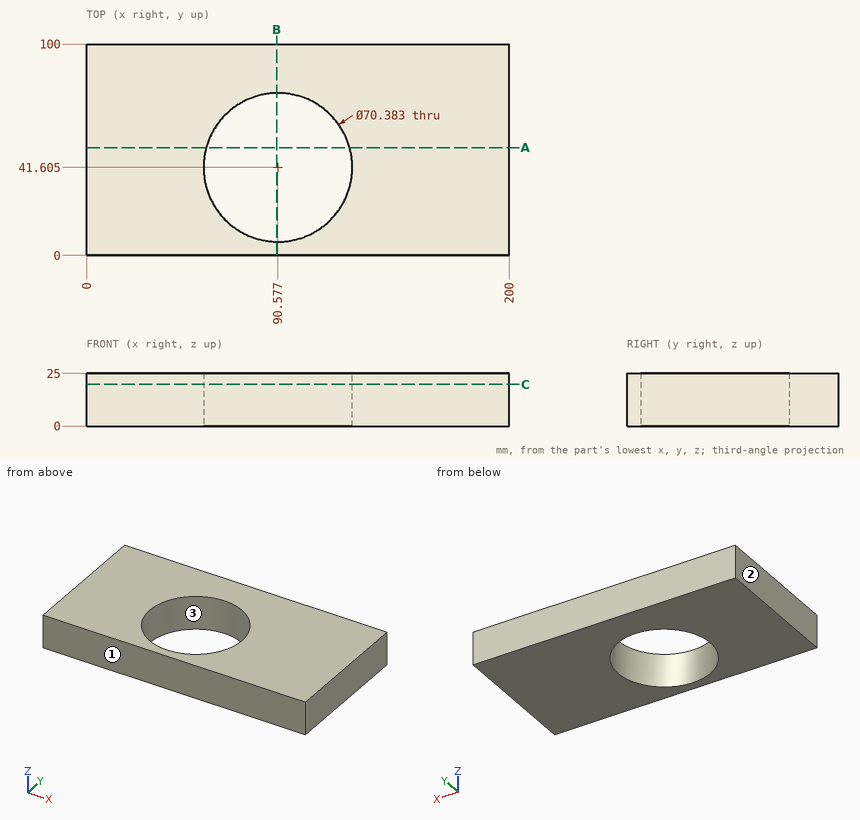
Could you check a few things on this drawing? It's one solid part, dimensions in mm from its lowest x, y, z. Give positions to 0.01 mm unless a question says otherwise; leave off trailing zeros. Order: outer loops, then holes, each group sorted by start corner. A loop starts at its lowest first (then second) coordinate and runs counter-clockwise, first axis right, second up. Notation, with made-up numbers: (34.5, -30) - (58.5, -30) arc R22 cw to (58.5, -24) - close; hole circle Ø5 at (21.5, 75.25). An arc over 180 degrees is marked (long way). One line per question, with ' | ' between items. Start each with the question number.
Item 1: I want a section at A-A on y = 51. Write out the boundary of the cut face in (x, z), then the cut area to 3 significant figures.
Item 2: I want a section at B-B on x = 90. Write out the boundary of the cut face in (y, z).
Item 3: I want a section at C-C on z = 19.75. Write out the boundary of the cut face in (x, y) (1 decimal).
Item 4: I need wall thicknesses on probe 1 along X at (y, z) = (57, 17.25); probe 2 along X at (y, z) = (16.5, 11.25) (1 decimal); probe 3 along Y at (x, z) = (118.5, 13) (1 decimal). Which ranges of each line are inside material? Lowest first, please. Write a range as [from, to].
Item 5: I'm going to push a flat-ended pin straight in: pin 1 Ø5 at (x, z) = (139.5, 5.5) entering from -Y. Where does the tip first touch, or does it pass through?
Item 6: Thinking about a two-plate mould opening in X: for the marked faces 1, 2 and 3, which applies, pulls with the +X half, pulls with the -X half, needs draft (parallel to the pull), parting line crosses it, or undercut?
Verdict:
1) outline: (0, 0) - (56.66, 0) - (56.66, 25) - (0, 25) - close; (124.49, 0) - (200, 0) - (200, 25) - (124.49, 25) - close | area: 3,300 mm^2
2) outline: (0, 0) - (6.42, 0) - (6.42, 25) - (0, 25) - close; (76.79, 0) - (100, 0) - (100, 25) - (76.79, 25) - close
3) outline: (0, 0) - (200, 0) - (200, 100) - (0, 100) - close; hole circle Ø70.4 at (90.6, 41.6)
4) probe 1: [0, 58.93], [122.22, 200] | probe 2: [0, 65.9], [115.2, 200] | probe 3: [0, 20.2], [63, 100]
5) pin 1: y = 0
6) face 1: needs draft | face 2: pulls with the -X half | face 3: undercut
